Source: CAD feature listing. Evaluate the final solid. Frame: model axes, mm. A direction names the side the tool comes from. Give positions to 0.01 mm unless a question says otherwise; leave off trailing zeros. Order: outer loops, then holes, each group sorted by start corner. A loop starts at its lowest first (then second) coordinate and runs counter-clockwise, first axis right, second up. Notation, with made-up numbers: M -39,17 L -8,17 A24 cw -8,52 Z; hole C 70.25,-15.75 d1. An arc over 180 degrees is marked long. Answer as a JSON object with one key per item and string values. Group by question number.
1. Set-up query: faces 1 (the flat face through (0, 0, 16)), 2 (the flat face through (14, 0, 12)). Return all of +Z, -Z, +X, -X, +Y, -Y with unobstructed straight access to the full face (end or side cutting, diameter ignored); none if empty.
2. Section query D-D (y = -20). Output: boundary loops of the cut face in (x, z).
3. Section query C-C (z = 14.75). Output: boundary loops of the cut face in (x, y), plus the area to 3 significant figures.
4. Section query A-A (y = 0). Output: boundary loops of the cut face in (x, z).
5. Pin query (flat end, axial travel): P1, Ø5, axis at x = 1.5, z = 4, coming from the -Y side; P2, Ø1.5, axis at x = 13, y = 25.5, coming from the +Z side; P3, Ø3, axis at x = 10.5, z = 7.5, coming from the +Y side. Return the tip coordinate at first contact, or that it passes through.
6. Material intervals for L1, parallel to Y at x = 0, z = 13; L2, parallel to Z at x = 16.5, y = 20; L3, parallel to Y at x = 27.5, z = 6.5, sorted ascending. Write a range as [from, to].
from build123d import *

# Parameters (mm, degrees)
SKETCH_01_WHEEL_PROFILE_R           = 32
PAD_02_WHEEL_DEPTH                  = 12
SKETCH_03_FRONTHUB_PROFILE_R        = 13.5
PAD_04_FRONTHUB_DEPTH               = 4
SKETCH_05_CENTER_SCREW_HOLE_R       = 1.2
POCKET_06_CENTER_SCREW_HOLE_DEPTH   = 18
SKETCH_07_SERVOHORN_POCKET_R        = 10.4
POCKET_08_SERVOHORN_POCKET_DEPTH    = 2.6
SKETCH_09_HORN_SCREW_HOLES_4X_R     = 1.1
POCKET_10_HORN_SCREW_HOLES_4X_DEPTH = 18
SKETCH_11_SPOKE_CUTOUTS_6X_R        = 4
POCKET_12_SPOKE_CUTOUTS_6X_DEPTH    = 18


with BuildPart() as part:
    # Sketch_01_Wheel_Profile → Pad_02_Wheel (new body)
    with BuildSketch(Plane.XY):
        Circle(SKETCH_01_WHEEL_PROFILE_R)
    extrude(amount=PAD_02_WHEEL_DEPTH)

    # Sketch_03_FrontHub_Profile → Pad_04_FrontHub (join)
    with BuildSketch(Plane.XY.offset(12)):
        Circle(SKETCH_03_FRONTHUB_PROFILE_R)
    extrude(amount=PAD_04_FRONTHUB_DEPTH)

    # Sketch_05_Center_Screw_Hole → Pocket_06_Center_Screw_Hole (cut)
    with BuildSketch(Plane.XY.offset(16)):
        Circle(SKETCH_05_CENTER_SCREW_HOLE_R)
    extrude(amount=POCKET_06_CENTER_SCREW_HOLE_DEPTH, mode=Mode.SUBTRACT)

    # Sketch_07_ServoHorn_Pocket → Pocket_08_ServoHorn_Pocket (cut)
    with BuildSketch(Plane.XY.offset(16)):
        Circle(SKETCH_07_SERVOHORN_POCKET_R)
    extrude(amount=POCKET_08_SERVOHORN_POCKET_DEPTH, mode=Mode.SUBTRACT)

    # Sketch_09_Horn_Screw_Holes_4x → Pocket_10_Horn_Screw_Holes_4x (cut)
    with BuildSketch(Plane.XY.offset(16)):
        with Locations((7.5, 0)):
            Circle(SKETCH_09_HORN_SCREW_HOLES_4X_R)
        with Locations((0, 7.5)):
            Circle(SKETCH_09_HORN_SCREW_HOLES_4X_R)
        with Locations((-7.5, 0)):
            Circle(SKETCH_09_HORN_SCREW_HOLES_4X_R)
        with Locations((0, -7.5)):
            Circle(SKETCH_09_HORN_SCREW_HOLES_4X_R)
    extrude(amount=POCKET_10_HORN_SCREW_HOLES_4X_DEPTH, mode=Mode.SUBTRACT)

    # Sketch_11_Spoke_Cutouts_6x → Pocket_12_Spoke_Cutouts_6x (cut)
    with BuildSketch(Plane.XY.offset(16)):
        with Locations((19.5, 0)):
            Circle(SKETCH_11_SPOKE_CUTOUTS_6X_R)
        with Locations((9.75, 16.887495)):
            Circle(SKETCH_11_SPOKE_CUTOUTS_6X_R)
        with Locations((-9.75, 16.887495)):
            Circle(SKETCH_11_SPOKE_CUTOUTS_6X_R)
        with Locations((-19.5, 0)):
            Circle(SKETCH_11_SPOKE_CUTOUTS_6X_R)
        with Locations((-9.75, -16.887495)):
            Circle(SKETCH_11_SPOKE_CUTOUTS_6X_R)
        with Locations((9.75, -16.887495)):
            Circle(SKETCH_11_SPOKE_CUTOUTS_6X_R)
    extrude(amount=POCKET_12_SPOKE_CUTOUTS_6X_DEPTH, mode=Mode.SUBTRACT)


solid = part.part
Answer sheet:
{
 "1": {"face 1": "+Z, +X, -X, +Y, -Y", "face 2": "+Z"},
 "2": {"outline": "M -24.98,0 L 24.98,0 L 24.98,12 L -24.98,12 Z"},
 "3": {"outline": "C 0,0 d27", "area": "573 mm^2"},
 "4": {"outline": "M -32,0 L 32,0 L 32,12 L 13.5,12 L 13.5,16 L -13.5,16 L -13.5,12 L -32,12 Z"},
 "5": {"P1": "y = -32", "P2": "z = 12", "P3": "y = 30.71"},
 "6": {"L1": "[-13.5, 13.5]", "L2": "[0, 12]", "L3": "[-16.36, 16.36]"}
}
